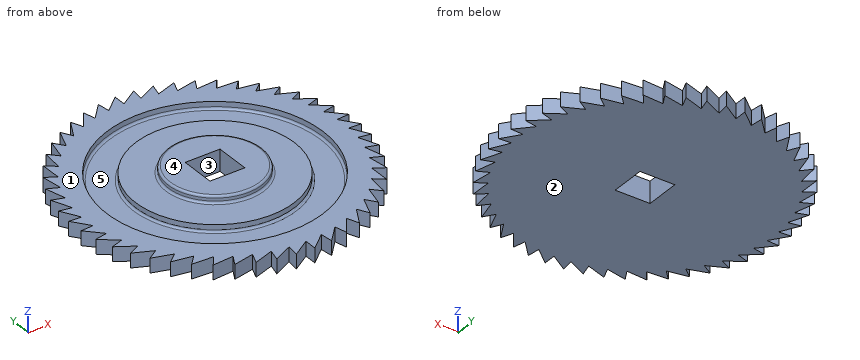
```python
from build123d import *

# Parameters (mm, degrees)
BOSS_EXTRUDE1_DEPTH = 2
CIRPATTERN1_COUNT   = 50
SKETCH3_W           = 4.842640688
SKETCH3_H           = 4.842640688
CUT_EXTRUDE2_DEPTH  = 3
SKETCH4_R           = 15
SKETCH4_R_2         = 11
CUT_EXTRUDE3_DEPTH  = 1
SKETCH5_R           = 6.5
SKETCH5_W           = 4.842640688
SKETCH5_H           = 4.842640688
BOSS_EXTRUDE2_DEPTH = 1
FILLET1_R           = 0.3


with BuildPart() as part:
    # Sketch2 → Boss-Extrude1 (new body)
    with BuildSketch(Plane.XY):
        with BuildLine():
            Line((0, -91), (0, -89))
            Line((0, -89), (-2.618249578, -91.196972255))
            ThreePointArc((-2.618249578, -91.196972255), (1.312824143, -125.950687458), (0, -91))
        make_face()
    boss_extrude1 = extrude(amount=-BOSS_EXTRUDE1_DEPTH)

    # CirPattern1: Boss-Extrude1 ×50 about axis
    cirpattern1_axis = Axis((0, -108.5, 0), (0, 0, 1))
    for i in range(1, CIRPATTERN1_COUNT):
        add(boss_extrude1.rotate(cirpattern1_axis, i * 360 / CIRPATTERN1_COUNT))

    # Sketch3 → Cut-Extrude2 (cut, through all)
    with BuildSketch(Plane.XY):
        with Locations((0, -108.5)):
            Rectangle(SKETCH3_W, SKETCH3_H)
    extrude(amount=-CUT_EXTRUDE2_DEPTH, mode=Mode.SUBTRACT)

    # Sketch4 → Cut-Extrude3 (cut)
    with BuildSketch(Plane.XY):
        with Locations((0, -108.5)):
            Circle(SKETCH4_R)
        with Locations((0, -108.5)):
            Circle(SKETCH4_R_2, mode=Mode.SUBTRACT)
    extrude(amount=-CUT_EXTRUDE3_DEPTH, mode=Mode.SUBTRACT)

    # Sketch5 → Boss-Extrude2 (add)
    with BuildSketch(Plane.XY):
        with Locations((0, -108.5)):
            Circle(SKETCH5_R)
        with Locations((0, -108.5)):
            Rectangle(SKETCH5_W, SKETCH5_H, mode=Mode.SUBTRACT)
    extrude(amount=BOSS_EXTRUDE2_DEPTH)

    # Fillet1
    fillet1_edges = [part.edges().sort_by_distance(p)[0] for p in [
        (-15, -108.5, -1),
        (-11, -108.5, -1),
        (-6.5, -108.5, 1),
        (-6.5, -108.5, 0),
    ]]
    fillet(fillet1_edges, radius=FILLET1_R)


solid = part.part
```
Build history of the part. All positions in model axes, mm. Face numbers are marked on the shaded views. A direction names the side the tool comes from. Coordinates: 2 decimals unless noted, no trailing zeros. Order: outer loops, then holes, each group sorted by start corner. A loop starts at its lowest first (then second) coordinate and runs counter-clockwise, first axis right, second up.
Item 1: Mould opens along Y. For the marked faces 4 and 5 say: released by +Y, released by -Y, zero draft, split by the parting line, or undercut.
Filled in:
face 4: zero draft
face 5: undercut
Item 2: Saw through at A-A on y = -108.5. List the corners of the cut face in (x, z).
Filled in:
outline: (-18.56, -2) - (-2.42, -2) - (-2.42, 1) - (-6.2, 1) arc R0.3 ccw to (-6.5, 0.7) - (-6.5, 0.3) arc R0.3 cw to (-6.8, 0) - (-11, 0) - (-11, -0.7) arc R0.3 cw to (-11.3, -1) - (-14.7, -1) arc R0.3 cw to (-15, -0.7) - (-15, 0) - (-18.56, 0) - close; (2.42, -2) - (18.56, -2) - (18.56, 0) - (15, 0) - (15, -0.7) arc R0.3 cw to (14.7, -1) - (11.3, -1) arc R0.3 cw to (11, -0.7) - (11, 0) - (6.8, 0) arc R0.3 cw to (6.5, 0.3) - (6.5, 0.7) arc R0.3 ccw to (6.2, 1) - (2.42, 1) - close
Item 3: Drill centre lines: L1, parallel to X at y = -109, z = -0.55; L2, parallel to Y at x = 2.5, z = -0.45; L3, parallel to Z at x = 14, y = -104.5. Where is each one in solid material? Low to high.
Filled in:
L1: x = -18.19 to -14.99, -10.99 to -2.42, 2.42 to 10.99, 14.99 to 18.93
L2: y = -127.79 to -123.29, -119.21 to -97.79, -93.71 to -90.74
L3: z = -2 to -1
Item 4: Tool access for the marked faces 1, 2 and 3: list every direction of +Z, -Z, +X, -X, +Y, -Y with a clear straight run to the whole face (end or side of a thin tool).
Filled in:
face 1: +Z
face 2: -Z, +X, -X, +Y, -Y
face 3: +Z, -Z
Item 5: Drop flat-ended pins along their axis: pin 1 Ø1.5 at (y, z) = (-114.5, 0.5) entering from +X; pin 2 Ø1.4 at (y, z) = (-90, -1) entering from +X; pin 3 Ø1.5 at (x, z) = (0.5, -1) entering from -Y. Give the stop position or say it passes through.
Filled in:
pin 1: stops at x = 18.55
pin 2: stops at x = 7.18
pin 3: stops at y = -128
